The model under review builds one solid part; all positions refer to its coordinate system, in mm. Face numbers are marked on the shaded views. A direction names the side the tool comes from. Coordinates: 2 decimals unless noted, no trailing zeros. Write each loop counter-clockwise with the first axis right and the second up, starting at its lowest first coordinate (ties: lowest second). Pieces come first, ordered by that corner, then holes. Notation, with made-up numbers: (39, 27.25) - (49, 27.25) arc R8 cw to (49, 40.25) - close; hole circle Ø7 at (-20.5, 13). An arc over 180 degrees is marked (long way). Put each result on its own line as item: value.
Autodesk Fusion 360 part; units mm, degrees
sketch "Esquisse1" plane through (0, 0, 0) normal (0, 0, 1) x (1, 0, 0)
  line L0 (-52.5, 35) -> (52.5, 35)
  line L1 (52.5, 35) -> (52.5, -35)
  line L2 (-52.5, -35) -> (-52.5, 35)
  line L3 (0, 1.75) -> (0, 22.5)
  line L4 (1.75, 0) -> (22.5, 0)
  line L5 (-23.5, -35) -> (-23.5, -87)
  line L6 (-23.5, -87) -> (23.5, -87)
  line L7 (23.5, -87) -> (23.5, -35)
  line L8 (52.5, -35) -> (23.5, -35)
  line L9 (-23.5, -35) -> (-52.5, -35)
  dimension "d1" = 105
  dimension "d2" = 70
  dimension "d25" = 52
  dimension "d26" = 47
extrude "Extrusion1" add sketch "Esquisse1" against normal blind 20
sketch "Esquisse3" plane through (0, 0, -20) normal (0, 0, -1) x (1, 0, 0)
  line L0 (-23.5, 35) -> (-52.5, 35)
  line L1 (-52.5, 35) -> (-52.5, -35)
  line L2 (-52.5, -35) -> (52.5, -35)
  line L3 (52.5, -35) -> (52.5, 35)
  line L4 (0, -1.75) -> (0, -22.5)
  line L5 (23.5, 87) -> (-23.5, 87)
  line L6 (-23.5, 87) -> (-23.5, 35)
  line L7 (52.5, 35) -> (23.5, 35)
  line L8 (23.5, 35) -> (23.5, 87)
  point P0 (-47, 28)
  point P1 (-23, 28)
  point P2 (-47, 10.2)
  point P3 (-23, 10.2)
  dimension "d7" = 24
  dimension "d8" = -17.8
  dimension "d16" = 47
hole "Perçage1" at (-47, -28, -20) at (-23, -28, -20) at (-23, -10.2, -20) at (-47, -10.2, -20) direction (0, 0, 1) diameter 5 depth 50 tip angle 118 counterbore diameter 8 counterbore depth 5
mirror "Symétrie miroir1" about plane through (0, 0, 0) normal (1, 0, 0) of "Perçage1"
mirror "Symétrie miroir2" about plane through (0, 0, 0) normal (0, 1, 0) of "Perçage1", "Symétrie miroir1"
sketch "Esquisse4" plane through (0, 0, -20) normal (0, 0, -1) x (1, 0, 0)
  line L0 (-23.5, 35) -> (-52.5, 35)
  line L1 (-52.5, 35) -> (-52.5, -35)
  line L2 (-52.5, -35) -> (52.5, -35)
  line L3 (52.5, -35) -> (52.5, 35)
  circle A0 centre (-40, 0) radius 4.075
  line L4 (23.5, 87) -> (-23.5, 87)
  line L5 (-23.5, 87) -> (-23.5, 35)
  line L6 (52.5, 35) -> (23.5, 35)
  line L7 (23.5, 35) -> (23.5, 87)
  circle A1 centre (23, -10.2) radius 4
  circle A2 centre (47, -28) radius 4
  circle A3 centre (23, -28) radius 4
  circle A4 centre (47, -10.2) radius 4
  circle A5 centre (-23, -10.2) radius 4
  circle A6 centre (-47, -28) radius 4
  circle A7 centre (-23, -28) radius 4
  circle A8 centre (-47, -10.2) radius 4
  circle A9 centre (23, 10.2) radius 4
  circle A10 centre (47, 28) radius 4
  circle A11 centre (23, 28) radius 4
  circle A12 centre (47, 10.2) radius 4
  circle A13 centre (-23, 10.2) radius 4
  circle A14 centre (-47, 28) radius 4
  circle A15 centre (-23, 28) radius 4
  circle A16 centre (-47, 10.2) radius 4
  dimension "d17" = 8.15
  dimension "d18" = 40
extrude "Extrusion2" cut sketch "Esquisse4" against normal blind 15 contours A0
mirror "Symétrie miroir3" about plane through (0, 0, 0) normal (1, 0, 0) of "Extrusion2"
sketch "Esquisse6" plane through (0, 0, -20) normal (0, 0, -1) x (1, 0, 0)
  circle A0 centre (40, 0) radius 4.075
  circle A1 centre (-40, 0) radius 4.075
  line L0 (23.5, 87) -> (-23.5, 87)
  line L1 (-23.5, 87) -> (-23.5, 35)
  line L2 (-23.5, 35) -> (-52.5, 35)
  line L3 (-52.5, 35) -> (-52.5, -35)
  line L4 (-52.5, -35) -> (52.5, -35)
  line L5 (52.5, -35) -> (52.5, 35)
  line L6 (52.5, 35) -> (23.5, 35)
  line L7 (23.5, 35) -> (23.5, 87)
  line L8 (-21.1, 77) -> (21.1, 77)
  line L9 (21.1, 77) -> (21.1, 34.8)
  line L10 (21.1, 34.8) -> (-21.1, 34.8)
  line L11 (-21.1, 34.8) -> (-21.1, 77)
  line L12 (0, -1.75) -> (0, -22.5)
  circle A2 centre (23, -10.2) radius 4
  circle A3 centre (47, -28) radius 4
  circle A4 centre (23, -28) radius 4
  circle A5 centre (47, -10.2) radius 4
  circle A6 centre (-23, -10.2) radius 4
  circle A7 centre (-47, -28) radius 4
  circle A8 centre (-23, -28) radius 4
  circle A9 centre (-47, -10.2) radius 4
  circle A10 centre (23, 10.2) radius 4
  circle A11 centre (47, 28) radius 4
  circle A12 centre (23, 28) radius 4
  circle A13 centre (47, 10.2) radius 4
  circle A14 centre (-23, 10.2) radius 4
  circle A15 centre (-47, 28) radius 4
  circle A16 centre (-23, 28) radius 4
  circle A17 centre (-47, 10.2) radius 4
  dimension "d27" = 42.2
  dimension "d28" = 42.2
  dimension "d29" = 10
extrude "Extrusion3" cut sketch "Esquisse6" against normal blind 12 contours L8 L9 L10 L11
sketch "Esquisse7" plane through (0, 0, -8) normal (0, 0, -1) x (1, 0, 0)
  line L0 (-21.1, 34.8) -> (21.1, 34.8)
  line L1 (21.1, 34.8) -> (21.1, 77)
  line L2 (21.1, 77) -> (-21.1, 77)
  line L3 (-21.1, 77) -> (-21.1, 34.8)
  circle A0 centre (0, 55.9) radius 11.1
  line L4 (-21.1, 77) -> (21.1, 77)
  line L5 (0, -1.75) -> (0, -22.5)
  dimension "d32" = 22.2
  dimension "d33" = 21.1
extrude "Extrusion4" cut sketch "Esquisse7" against normal blind 2.5 contours A0
sketch "Esquisse8" plane through (0, 0, -5.5) normal (0, 0, -1) x (1, 0, 0)
  circle A0 centre (0, 55.9) radius 11.1
  circle A1 centre (0, 55.9) radius 4
  dimension "d36" = 8
extrude "Extrusion5" cut sketch "Esquisse8" against normal blind 9 contours A1
sketch "Esquisse9" plane through (0, 0, -20) normal (0, 0, -1) x (1, 0, 0)
  line L0 (21.1, 77) -> (21.1, 34.8)
  line L1 (21.1, 34.8) -> (-21.1, 34.8)
  line L2 (-21.1, 34.8) -> (-21.1, 77)
  line L3 (-21.1, 77) -> (21.1, 77)
  circle A0 centre (40, 0) radius 4.075
  circle A1 centre (-40, 0) radius 4.075
  line L4 (23.5, 87) -> (-23.5, 87)
  line L5 (-23.5, 87) -> (-23.5, 35)
  line L6 (-23.5, 35) -> (-52.5, 35)
  line L7 (-52.5, 35) -> (-52.5, -35)
  line L8 (-52.5, -35) -> (52.5, -35)
  line L9 (52.5, -35) -> (52.5, 35)
  line L10 (52.5, 35) -> (23.5, 35)
  line L11 (23.5, 35) -> (23.5, 87)
  circle A2 centre (0, 0) radius 11.15
  circle A3 centre (23, -10.2) radius 4
  circle A4 centre (47, -28) radius 4
  circle A5 centre (23, -28) radius 4
  circle A6 centre (47, -10.2) radius 4
  circle A7 centre (-23, -10.2) radius 4
  circle A8 centre (-47, -28) radius 4
  circle A9 centre (-23, -28) radius 4
  circle A10 centre (-47, -10.2) radius 4
  circle A11 centre (23, 10.2) radius 4
  circle A12 centre (47, 28) radius 4
  circle A13 centre (23, 28) radius 4
  circle A14 centre (47, 10.2) radius 4
  circle A15 centre (-23, 10.2) radius 4
  circle A16 centre (-47, 28) radius 4
  circle A17 centre (-23, 28) radius 4
  circle A18 centre (-47, 10.2) radius 4
  dimension "d39" = 22.3
extrude "Extrusion6" cut sketch "Esquisse9" against normal blind 8 contours A2
sketch "Esquisse10" plane through (0, 0, 0) normal (0, 0, 1) x (-1, 0, 0)
  circle A0 centre (-23, -10.2) radius 2.5
  circle A1 centre (-47, -28) radius 2.5
  circle A2 centre (-23, -28) radius 2.5
  circle A3 centre (-47, -10.2) radius 2.5
  circle A4 centre (23, -10.2) radius 2.5
  circle A5 centre (47, -28) radius 2.5
  circle A6 centre (23, -28) radius 2.5
  circle A7 centre (47, -10.2) radius 2.5
  circle A8 centre (-23, 10.2) radius 2.5
  circle A9 centre (-47, 28) radius 2.5
  circle A10 centre (-23, 28) radius 2.5
  circle A11 centre (-47, 10.2) radius 2.5
  circle A12 centre (23, 10.2) radius 2.5
  circle A13 centre (47, 28) radius 2.5
  circle A14 centre (23, 28) radius 2.5
  circle A15 centre (47, 10.2) radius 2.5
  line L0 (23.5, 87) -> (-23.5, 87)
  line L1 (-23.5, 87) -> (-23.5, 35)
  line L2 (-23.5, 35) -> (-52.5, 35)
  line L3 (-52.5, 35) -> (-52.5, -35)
  line L4 (-52.5, -35) -> (52.5, -35)
  line L5 (52.5, -35) -> (52.5, 35)
  line L6 (52.5, 35) -> (23.5, 35)
  line L7 (23.5, 35) -> (23.5, 87)
  circle A16 centre (0, 0) radius 11.15
  circle A17 centre (0, 55.9) radius 4
  dimension "d42" = 22.3
extrude "Extrusion7" cut sketch "Esquisse10" against normal blind 8 contours A16
sketch "Esquisse11" plane through (0, 0, -12) normal (0, 0, -1) x (1, 0, 0)
  circle A0 centre (0, 0) radius 11.15
  circle A1 centre (0, 0) radius 4.5
  dimension "d45" = 9
extrude "Extrusion8" cut sketch "Esquisse11" against normal blind 15 contours A1
sketch "Esquisse12" plane through (0, 0, -8) normal (0, 0, -1) x (1, 0, 0)
  circle A0 centre (0, 55.9) radius 11.1
  line L0 (-21.1, 34.8) -> (21.1, 34.8)
  line L1 (21.1, 34.8) -> (21.1, 77)
  line L2 (21.1, 77) -> (-21.1, 77)
  line L3 (-21.1, 77) -> (-21.1, 34.8)
  point P0 (-15.5, 71.4)
  point P1 (15.5, 71.4)
  point P2 (-15.5, 40.4)
  point P3 (15.5, 40.4)
  dimension "d48" = 15.5
  dimension "d49" = 15.5
  dimension "d52" = 31
  dimension "d53" = -31
hole "Perçage2" at (-15.5, -71.4, -8) at (15.5, -71.4, -8) at (15.5, -40.4, -8) at (-15.5, -40.4, -8) direction (0, 0, 1) diameter 4 depth 50 tip angle 118
sketch "Esquisse13" plane through (0, 0, 0) normal (0, 0, 1) x (-1, 0, 0)
  circle A0 centre (-15.5, 40.4) radius 2
  circle A1 centre (15.5, 71.4) radius 2
  circle A2 centre (-15.5, 71.4) radius 2
  circle A3 centre (15.5, 40.4) radius 2
  circle A4 centre (0, 0) radius 11.15
  circle A5 centre (0, 55.9) radius 4
  circle A6 centre (-23, -10.2) radius 2.5
  circle A7 centre (-47, -28) radius 2.5
  circle A8 centre (-23, -28) radius 2.5
  circle A9 centre (-47, -10.2) radius 2.5
  circle A10 centre (23, -10.2) radius 2.5
  circle A11 centre (47, -28) radius 2.5
  circle A12 centre (23, -28) radius 2.5
  circle A13 centre (47, -10.2) radius 2.5
  circle A14 centre (-23, 10.2) radius 2.5
  circle A15 centre (-47, 28) radius 2.5
  circle A16 centre (-23, 28) radius 2.5
  circle A17 centre (-47, 10.2) radius 2.5
  circle A18 centre (23, 10.2) radius 2.5
  circle A19 centre (47, 28) radius 2.5
  circle A20 centre (23, 28) radius 2.5
  circle A21 centre (47, 10.2) radius 2.5
  line L0 (23.5, 87) -> (-23.5, 87)
  line L1 (-23.5, 87) -> (-23.5, 35)
  line L2 (-23.5, 35) -> (-52.5, 35)
  line L3 (-52.5, 35) -> (-52.5, -35)
  line L4 (-52.5, -35) -> (52.5, -35)
  line L5 (52.5, -35) -> (52.5, 35)
  line L6 (52.5, 35) -> (23.5, 35)
  line L7 (23.5, 35) -> (23.5, 87)
  point P0 (11, -30)
  dimension "d57" = 30
  dimension "d58" = 11
hole "Perçage3" at (-11, 30, 0) direction (0, 0, -1) diameter 4.5 depth 50 tip angle 118
mirror "Symétrie miroir4" about plane through (0, 0, 0) normal (1, 0, 0) of "Perçage3"
pattern_linear "Réseau R1" count 2 spacing 110.5 along (0, -1, 0) of "Symétrie miroir4", "Perçage3"
sketch "Esquisse14" plane through (0, 0, 0) normal (0, 0, 1) x (-1, 0, 0)
  circle A0 centre (-11, 80.5) radius 2.25
  circle A1 centre (11, 80.5) radius 2.25
  circle A2 centre (-11, -30) radius 2.25
  circle A3 centre (11, -30) radius 2.25
  circle A4 centre (-15.5, 40.4) radius 2
  circle A5 centre (15.5, 71.4) radius 2
  circle A6 centre (-15.5, 71.4) radius 2
  circle A7 centre (15.5, 40.4) radius 2
  circle A8 centre (0, 0) radius 11.15
  circle A9 centre (0, 55.9) radius 4
  circle A10 centre (-23, -10.2) radius 2.5
  circle A11 centre (-47, -28) radius 2.5
  circle A12 centre (-23, -28) radius 2.5
  circle A13 centre (-47, -10.2) radius 2.5
  circle A14 centre (23, -10.2) radius 2.5
  circle A15 centre (47, -28) radius 2.5
  circle A16 centre (23, -28) radius 2.5
  circle A17 centre (47, -10.2) radius 2.5
  circle A18 centre (-23, 10.2) radius 2.5
  circle A19 centre (-47, 28) radius 2.5
  circle A20 centre (-23, 28) radius 2.5
  circle A21 centre (-47, 10.2) radius 2.5
  circle A22 centre (23, 10.2) radius 2.5
  circle A23 centre (47, 28) radius 2.5
  circle A24 centre (23, 28) radius 2.5
  circle A25 centre (47, 10.2) radius 2.5
  line L0 (23.5, 87) -> (-23.5, 87)
  line L1 (-23.5, 87) -> (-23.5, 35)
  line L2 (-23.5, 35) -> (-52.5, 35)
  line L3 (-52.5, 35) -> (-52.5, -35)
  line L4 (-52.5, -35) -> (52.5, -35)
  line L5 (52.5, -35) -> (52.5, 35)
  line L6 (52.5, 35) -> (23.5, 35)
  line L7 (23.5, 35) -> (23.5, 87)
  circle A26 centre (0, -20) radius 1.3
  line L8 (-20, 0) -> (-2.5, 0)
  dimension "d70" = 2.6
  dimension "d71" = 20
extrude "Extrusion9" cut sketch "Esquisse14" against normal blind 24 contours A26
mirror "Symétrie miroir5" about plane through (0, 0, 0) normal (0, 1, 0) of "Extrusion9"
fillet "Congé1" radius 5 8 edges at (-52.5, 35, -10) (52.5, 35, -10) (52.5, -35, -10) (23.5, -87, -10) (-23.5, -87, -10) (-23.5, -35, -10) (23.5, -35, -10) (-52.5, -35, -10)
equation "d16 = ( ( 70 / 2 ) * 1 mm ) + 12 mm"
equation "d32 = ( 11.10 * 2 ) * 1 mm"
equation "d33 = ( 42.2 / 2 ) * 1 mm"
equation "d48 = ( 31 / 2 ) * 1 mm"
equation "d49 = ( 31 / 2 ) * 1 mm"
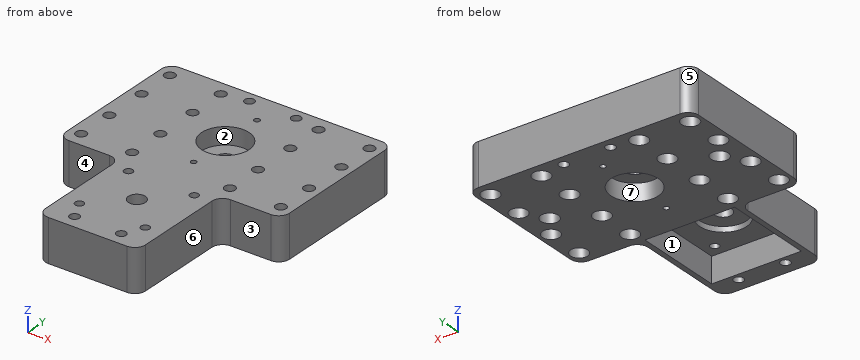
1. For pin 1 Ø6 at (x, y) = (23, 28) entering from +Z; pin 2 Ø3 at (x, z) = (-40.5, -7.5) entering from -Y; pin 3 Ø4 at (x, y) = (22, 29) entering from -Z; pin 4 Ø1 at (y, z) = (-47.5, -9) entering from +X, all flat-tipped, find the tip position at first contact; note any pin that passes through.
Determined:
pin 1: stops at z = 0
pin 2: stops at y = -35
pin 3: stops at z = -15
pin 4: stops at x = 23.5
2. Consider section C-C on z = -18. Give the number of separate pieces and of enclosed holes in the cut face, plus the area to 3 significant figures.
Determined:
separate pieces: 1
enclosed holes: 26
area: 6,620 mm^2
3. Consider section A-A on y = 20. State the section outline as (x, z) points, plus the area to 3 significant figures.
Determined:
outline: (-52.5, -20) - (-1.3, -20) - (-1.3, 0) - (-52.5, 0) - close; (1.3, -20) - (52.5, -20) - (52.5, 0) - (1.3, 0) - close
area: 2,050 mm^2
4. Consider section B-B on x = 15.5. State the section outline as (y, z) points.
Determined:
outline: (-87, -20) - (-77, -20) - (-77, -8) - (-73.4, -8) - (-73.4, 0) - (-87, 0) - close; (-69.4, -8) - (-42.4, -8) - (-42.4, 0) - (-69.4, 0) - close; (-38.4, -8) - (-34.8, -8) - (-34.8, -20) - (35, -20) - (35, 0) - (-38.4, 0) - close
5. To check wall thickness, follow probe 1 along Y at (x, z) = (15.5, -3); probe 2 along X at (y, z) = (-10.2, -18.5); probe 3 along Y at (x, z) = (0, -4.25). State the ranges of each line that lie inside material, in increasing order.
Determined:
probe 1: y = -87 to -73.4, -69.4 to -42.4, -38.4 to 35
probe 2: x = -52.5 to -51, -43 to -27, -19 to -4.5, 4.5 to 19, 27 to 43, 51 to 52.5
probe 3: y = -87 to -59.9, -51.9 to -21.3, -18.7 to -11.15, 11.15 to 18.7, 21.3 to 35
6. Consider section D-D on y = 0. State the section outline as (x, z) points (3 decimals), plus the area to 3 significant figures.
Determined:
outline: (-52.5, -20) - (-44.075, -20) - (-44.075, -5) - (-35.925, -5) - (-35.925, -20) - (-11.15, -20) - (-11.15, -12) - (-4.5, -12) - (-4.5, -8) - (-11.15, -8) - (-11.15, 0) - (-52.5, 0) - close; (4.5, -12) - (11.15, -12) - (11.15, -20) - (35.925, -20) - (35.925, -5) - (44.075, -5) - (44.075, -20) - (52.5, -20) - (52.5, 0) - (11.15, 0) - (11.15, -8) - (4.5, -8) - close
area: 1,460 mm^2
7. The part is to be moulded in two halves that separate along Y. For the marked faces 5, 6 and 7, say which applies: +Y half, -Y half, draft (parallel to the pull), parting line (faces both ways), or undercut.
Determined:
face 5: +Y half
face 6: draft
face 7: undercut
8. Machinability: for the marked faces 1, 2, 3 and 4, which of the approach directions +Z, -Z, +X, -X, +Y, -Y give a long, thin tool a straight path to every point of the face, cutting with its end or side? Answer none if there is none.
Determined:
face 1: -Z
face 2: +Z
face 3: +Z, -Z, +X, -Y
face 4: +Z, -Z, -X, -Y
